Build history of the part. All positions in model axes, mm. A direction names the side the tool comes from. Round coordinates to 2 decimals unless told otherwise and drop trailing zeros. Order: outer loops, then holes, each group sorted by start corner. A loop starts at its lowest first (then second) coordinate and runs counter-clockwise, first axis right, second up. Notation, with made-up numbers: (35.25, -11) -> (42.25, -11) arc R33 ccw to (42.25, 28) -> close; hole circle Ø7 at (20, 52). An arc over 180 degrees is marked (long way). Write item = value, one per line.
from build123d import *

# Parameters (mm, degrees)
F0_R     = 11
F1_DEPTH = 20


with BuildPart() as f1:
    # F0 (on Front) → F1 (new body)
    with BuildSketch(Plane.XZ):
        Polygon((0, 200), (0, 0), (200, 0), (200, 100), (300, 100), (300, 0), (500, 0), (500, 200), align=None)
        with Locations((40, 160)):
            Circle(F0_R, mode=Mode.SUBTRACT)
        with Locations((460, 160)):
            Circle(F0_R, mode=Mode.SUBTRACT)
    extrude(amount=F1_DEPTH)


solid = f1.part
Q1. Cut at C-C, the plane x = 40. List the corners of the cut face in (y, z).
Check values:
outline = (-20, 0) -> (0, 0) -> (0, 149) -> (-20, 149) -> close; (-20, 171) -> (0, 171) -> (0, 200) -> (-20, 200) -> close
Q2. Cut at D-D, the plane z = 160. List the corners of the cut face in (x, y).
Check values:
outline = (0, -20) -> (29, -20) -> (29, 0) -> (0, 0) -> close; (51, -20) -> (449, -20) -> (449, 0) -> (51, 0) -> close; (471, -20) -> (500, -20) -> (500, 0) -> (471, 0) -> close
Q3. Cut at B-B, the plane z = 58.5. List the corners of the cut face in (x, y).
Check values:
outline = (0, -20) -> (200, -20) -> (200, 0) -> (0, 0) -> close; (300, -20) -> (500, -20) -> (500, 0) -> (300, 0) -> close
Q4. Cut at A-A, the plane y = -9.5. List the corners of the cut face in (x, z), and give its area (3 significant figures).
Check values:
outline = (0, 0) -> (200, 0) -> (200, 100) -> (300, 100) -> (300, 0) -> (500, 0) -> (500, 200) -> (0, 200) -> close; hole circle Ø22 at (40, 160); hole circle Ø22 at (460, 160)
area = 89,200 mm²
Q5. Which spindle directions (+Z, -Z, +X, -X, +Y, -Y) get a long thin tool onto all of the face, cutting with end or side? Do faces 1 (the face through (99, -10, 0)), 2 (the face through (200, -10, 49)). Say none if no direction does.
Check values:
face_1 = -Z, +X, -X, +Y, -Y
face_2 = -Z, +Y, -Y
Q6. Probe probe 1 along X at (y, z) = (-8.25, 75.5); probe 2 along Z at (x, y) = (40, -7.25). List the from-to ranges inside material, lowest first.
Check values:
probe_1 = 0 to 200, 300 to 500
probe_2 = 0 to 149, 171 to 200
Q7. Mould opens along X. For faces 3 (the face through (399, -10, 0)), 4 (the face through (500, -10, 99)), 5 (the face through (249, -10, 100)) say: released by +X, released by -X, zero draft, split by the parting line, or undercut.
Check values:
face_3 = zero draft
face_4 = released by +X
face_5 = undercut
